```python
from build123d import *

# Parameters (mm, degrees)
SKETCH_1_W          = 20
SKETCH_1_H          = 20
EXTRUDE_1_DEPTH     = 50
SKETCH_2_R          = 2.5
CUT_EXTRUDE_1_DEPTH = 14
SKETCH_3_R          = 2.5
CUT_EXTRUDE_2_DEPTH = 14


with BuildPart() as part:
    # 草图1 → 凸台-拉伸1 (new body)
    with BuildSketch(Plane.XY):
        with Locations((10, 10)):
            Rectangle(SKETCH_1_W, SKETCH_1_H)
    extrude(amount=EXTRUDE_1_DEPTH)

    # 草图2 → 切除-拉伸1 (cut)
    with BuildSketch(Plane(origin=(20, 0, 0), x_dir=(0, 0, -1), z_dir=(1, 0, 0))):
        with Locations((-10, 10)):
            Circle(SKETCH_2_R)
        with Locations((-40, 10)):
            Circle(SKETCH_2_R)
    extrude(amount=-CUT_EXTRUDE_1_DEPTH, mode=Mode.SUBTRACT)

    # 草图3 → 切除-拉伸2 (cut)
    with BuildSketch(Plane(origin=(0, 20, 0), x_dir=(1, 0, 0), z_dir=(0, 1, 0))):
        with Locations(Location((10, -20, 0), (0, 0, 270))):
            Circle(SKETCH_3_R)
        with Locations(Location((10, -30, 0), (0, 0, 270))):
            Circle(SKETCH_3_R)
    extrude(amount=-CUT_EXTRUDE_2_DEPTH, mode=Mode.SUBTRACT)


solid = part.part
```
Can you work these out from the model? Positions are in its coordinate system, mm. A direction names the side the tool comes from. Round coordinates to 2 decimals unless told otherwise and drop trailing zeros. Loops run counter-clockwise (first coordinate to the right, second up) from the corner with the lowest first, then second, coordinate; pieces in that order, holes last. Notation, with made-up numbers: (2.5, 74.25) -> (60.5, 74.25) arc R21 ccw to (60.5, 79.25) -> close; hole circle Ø11 at (-30, 70). An arc over 180 degrees is marked (long way). Answer in a Markdown table with one row per item.
Item 1: Will this pin go through, and if not, where does the flat tip stop? P1, Ø2.5, axis at y = 9, z = 40.5, coming from the +X side.
Answer block:
| item | result |
|---|---|
| P1 | x = 6 |
Item 2: We'd pull the mould along Z, two halves only. Please class faces 4 (the flat face through (10, 10, 50)), 5 (the cylindrical face through (13.1, 9.04, 37.69)), 6 (the flat face through (10, 0, 25)): released by +Z, released by -Z, zero draft, split by the parting line, or undercut.
Answer block:
| item | result |
|---|---|
| face 4 | released by +Z |
| face 5 | undercut |
| face 6 | zero draft |
Item 3: Suppose I cut it at C-C, the plane x = 16.5. List the corners of the cut face in (y, z) for me.
Answer block:
| item | result |
|---|---|
| outline | (0, 0) -> (20, 0) -> (20, 50) -> (0, 50) -> close; hole circle Ø5 at (10, 10); hole circle Ø5 at (10, 40) |
Item 4: Suppose I cut it at A-A, the plane y = 17.75. List the corners of the cut face in (x, z) for me.
Answer block:
| item | result |
|---|---|
| outline | (0, 0) -> (20, 0) -> (20, 50) -> (0, 50) -> close; hole circle Ø5 at (10, 20); hole circle Ø5 at (10, 30) |
Item 5: On a 3-axis mill with a long thin cutter (end or side, diameter ignored), from which of +Z, -Z, +X, -X, +Y, -Y can I reach the whole of each face in a straight line? I mean faces 1 (the flat face through (6, 10, 40)), 2 (the flat face through (10, 6, 20)), 3 (the flat face through (0, 10, 25)). Say none if no direction works.
Answer block:
| item | result |
|---|---|
| face 1 | +X |
| face 2 | +Y |
| face 3 | +Z, -Z, -X, +Y, -Y |
Item 6: If I drill on probe 1 along Z at (x, y) = (9.75, 13); probe 2 along Y at (x, z) = (15.5, 10), over which ranges is the centre line in solid material (lowest first)?
Answer block:
| item | result |
|---|---|
| probe 1 | 0 to 17.51, 22.49 to 27.51, 32.49 to 50 |
| probe 2 | 0 to 7.5, 12.5 to 20 |
Item 7: Suppose I cut it at D-D, the plane z = 39. List the corners of the cut face in (x, y) for me.
Answer block:
| item | result |
|---|---|
| outline | (0, 0) -> (20, 0) -> (20, 7.71) -> (6, 7.71) -> (6, 12.29) -> (20, 12.29) -> (20, 20) -> (0, 20) -> close |
Item 8: Suppose I cut it at B-B, the plane z = 30. List the corners of the cut face in (x, y) for me, plus the area to 3 significant figures.
Answer block:
| item | result |
|---|---|
| outline | (0, 0) -> (20, 0) -> (20, 20) -> (12.5, 20) -> (12.5, 6) -> (7.5, 6) -> (7.5, 20) -> (0, 20) -> close |
| area | 330 mm² |
